```python
from build123d import *

# Parameters (mm, degrees)
EXTRUDE_1_DEPTH          = 10
CUT_EXTRUDE_1_DEPTH      = 53.855703508
CUT_EXTRUDE_1_DEPTH_BACK = 53.855703508
SKETCH_2_R               = 1.5
CUT_EXTRUDE_2_DEPTH      = 53.855703649
CUT_EXTRUDE_2_DEPTH_BACK = 53.855703649
SKETCH_3_R               = 5


with BuildPart() as part:
    # 草图1 → 凸台-拉伸1 (new body)
    with BuildSketch(Plane.XY):
        with BuildLine():
            ThreePointArc((-5.592370399, 49.686269666), (-10.344117547, 48.918291386), (-15, 47.696960071))
            Line((-15, 47.696960071), (-15, -47.696960071))
            ThreePointArc((-15, -47.696960071), (-10.344117547, -48.918291386), (-5.592370399, -49.686269666))
            Line((-5.592370399, -49.686269666), (-3.031088913, -45.25))
            ThreePointArc((-3.031088913, -45.25), (0, -43.5), (3.031088913, -45.25))
            Line((3.031088913, -45.25), (5.592370399, -49.686269666))
            ThreePointArc((5.592370399, -49.686269666), (10.344117547, -48.918291386), (15, -47.696960071))
            Line((15, -47.696960071), (15, 47.696960071))
            ThreePointArc((15, 47.696960071), (10.344117547, 48.918291386), (5.592370399, 49.686269666))
            Line((5.592370399, 49.686269666), (3.031088913, 45.25))
            ThreePointArc((3.031088913, 45.25), (0, 43.5), (-3.031088913, 45.25))
            Line((-3.031088913, 45.25), (-5.592370399, 49.686269666))
        make_face()
    extrude(amount=EXTRUDE_1_DEPTH)

    # 草图2 → 切除-拉伸1 (cut, two sides: drawn at the far end of the back side and taken through both)
    with BuildSketch(Plane(origin=(0, 0, 0), x_dir=(1, 0, 0), z_dir=(0, 1, 0)).offset(-CUT_EXTRUDE_1_DEPTH_BACK)):
        with Locations(Location((-10, -5, 0), (0, 0, 270))):
            Circle(SKETCH_2_R)
        with Locations(Location((10, -5, 0), (0, 0, 270))):
            Circle(SKETCH_2_R)
    extrude(amount=CUT_EXTRUDE_1_DEPTH + CUT_EXTRUDE_1_DEPTH_BACK, mode=Mode.SUBTRACT)

    # 草图3 → 切除-拉伸2 (cut, two sides: drawn at the far end of the back side and taken through both)
    with BuildSketch(Plane.XY.offset(10).offset(-CUT_EXTRUDE_2_DEPTH_BACK)):
        Circle(SKETCH_3_R)
    extrude(amount=CUT_EXTRUDE_2_DEPTH + CUT_EXTRUDE_2_DEPTH_BACK, mode=Mode.SUBTRACT)


solid = part.part
```
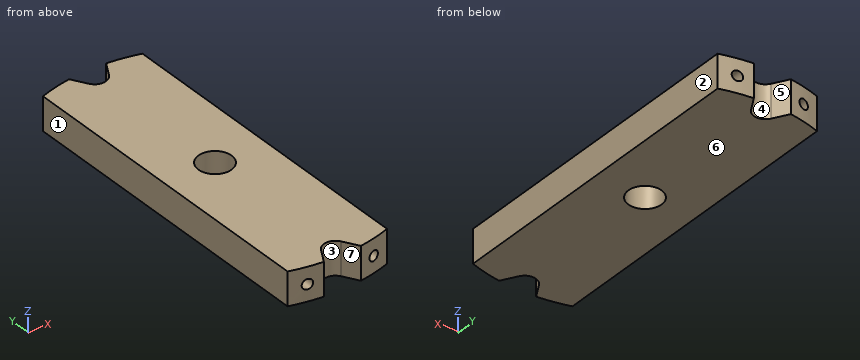
Here's how the part is built. I have some questions about the finished solid (model axes, mm). Face numbers are marked on the shaded views. A direction names the side the tool comes from. Give positions to 0.01 mm unless a question says otherwise; leave off trailing zeros. Order: outer loops, then holes, each group sorted by start corner. A loop starts at its lowest first (then second) coordinate and runs counter-clockwise, first axis right, second up. Notation, with made-up numbers: M 75,20 L 90,20 A15 cw 90,25 Z; hole C 14,83.25 d7. An arc over 180 degrees is marked long. Use a Markdown table: item, result. Add a question column.
1. For pin 1 Ø4 at (x, z) = (9.5, 1.5) entering from -Y; pin 2 Ø4 at (x, z) = (-3, 8) entering from +Y; pin 3 Ø2.5 at (x, z) = (-10, 5) entering from +Y, each with a flat end and sliding along its axis, tell me the tip position at first contact or that it passes through.
2. Suppose I cut it at B-B (z = 1.75). List the corners of the cut face in (x, y) for me, and give its area (3 significant figures).
3. On a 3-axis mill with a long thin cutter (end or side, diameter ignored), from which of +Z, -Z, +X, -X, +Y, -Y can I reach the whole of each face in a straight line? I mean the marked faces 5, 6 and 7. Say none if no direction works.
4. Suppose I cut it at C-C (x = 0). List the corners of the cut face in (y, z) for me, and give its area (3 significant figures).
5. If we mould it in two halves opening along X, with no side actions, what happens to the marked faces 1, 2, 3 and 4? For each: +X half, -X half, draft (parallel to the pull), parting line (faces both ways), or undercut.
6. Suppose I cut it at D-D (y = -18). List the corners of the cut face in (x, z) for me.
7. I need wall thicknesses on probe 1 along X at (y, z) = (13.5, 5); probe 2 along Z at (x, y) = (10, -11); probe 3 along X at (y, z) = (0, 7.25). Which ranges of each line are inside material? Lowest first, please. Write a range as from..to.
8. Suppose I cut it at A-A (y = 0). List the corners of the cut face in (x, z) for me.
Results list:
| question | item | result |
|---|---|---|
| 1 | pin 1 | stops at y = -49.43 |
| 1 | pin 2 | stops at y = 48.66 |
| 1 | pin 3 | passes through |
| 2 | outline | M -15,-47.7 A50 ccw -5.59,-49.69 L -3.03,-45.25 A3.5 cw 3.03,-45.25 L 5.59,-49.69 A50 ccw 15,-47.7 L 15,47.7 A50 ccw 5.59,49.69 L 3.03,45.25 A3.5 cw -3.03,45.25 L -5.59,49.69 A50 ccw -15,47.7 Z; hole C 0,0 d10 |
| 2 | area | 2,780 mm² |
| 3 | face 5 | +Z, -Z, +Y |
| 3 | face 6 | -Z, +X, -X, +Y, -Y |
| 3 | face 7 | +Z, -Z, -Y |
| 4 | outline | M -43.5,0 L -5,0 L -5,10 L -43.5,10 Z; M 5,0 L 43.5,0 L 43.5,10 L 5,10 Z |
| 4 | area | 770 mm² |
| 5 | face 1 | -X half |
| 5 | face 2 | +X half |
| 5 | face 3 | undercut |
| 5 | face 4 | undercut |
| 6 | outline | M -15,0 L 15,0 L 15,10 L -15,10 Z; hole C -10,5 d3; hole C 10,5 d3 |
| 7 | probe 1 | x = -15..-11.5, -8.5..8.5, 11.5..15 |
| 7 | probe 2 | z = 0..3.5, 6.5..10 |
| 7 | probe 3 | x = -15..-5, 5..15 |
| 8 | outline | M -15,0 L -5,0 L -5,10 L -15,10 Z; M 5,0 L 15,0 L 15,10 L 5,10 Z; hole C -10,5 d3; hole C 10,5 d3 |
